Work out the finished part from the listing and answer in its coordinate system (mm). A direction names the side the tool comes from. Give positions to 0.01 mm unless a question says otherwise; leave off trailing zeros. Order: outer loops, then holes, each group sorted by start corner. A loop starts at its lowest first (then second) coordinate and runs counter-clockwise, first axis right, second up. Notation, with made-up numbers: (48.5, 87.25) - (57.5, 87.25) arc R26 cw to (57.5, 122.25) - close; hole circle Ø7 at (29.25, 77). An arc over 180 degrees is marked (long way). Write each question's results on one line, items separated by ' | '.
from build123d import *

# Parameters (mm, degrees)
F0_W     = 19.05
F0_H     = 19.05
F0_W_2   = 15.875
F0_H_2   = 15.875
F1_DEPTH = 40
F3_DEPTH = 9.526
F4_DEPTH = 9.526
F5_R     = 3
F6_DEPTH = 9.526


with BuildPart() as f1:
    # F0 (on Front) → F1 (new body)
    with BuildSketch(Plane.XZ):
        Rectangle(F0_W, F0_H)
        Rectangle(F0_W_2, F0_H_2, mode=Mode.SUBTRACT)
    extrude(amount=F1_DEPTH)

    # F2 (on Top) → F3 (cut, through all)
    with BuildSketch(Plane.XY):
        Polygon((9.525, 0), (-9.525, 0), (-9.525, -19.05), align=None)
    extrude(amount=-F3_DEPTH, mode=Mode.SUBTRACT)

    # F2 (on Top) → F4 (cut, through all)
    with BuildSketch(Plane.XY):
        Polygon((9.525, 0), (-9.525, 0), (-9.525, -19.05), align=None)
    extrude(amount=F4_DEPTH, mode=Mode.SUBTRACT)

    # F5 (on Right) → F6 (cut, through all)
    with BuildSketch(Plane.YZ):
        with Locations((-32.75, 0)):
            Circle(F5_R)
    extrude(amount=-F6_DEPTH, mode=Mode.SUBTRACT)


solid = f1.part
1. Straight lines are drawn through the part: line 1 (X direction, y = -24, z = 0.5) (1 decimal); line 2 (Z direction, x = -8.5, y = -32.75) (3 decimals). For each, find the intervals that lie inside material, in ascending order. Write a range as [from, to].
Answer list:
line 1: [-9.5, -7.9], [7.9, 9.5] | line 2: [-9.525, -3], [3, 9.525]
2. A tool of negligible diameter and unlimited length cuts with its end or side. For faces 1 (the face through (-9, -40, 0)), 2 (the face through (0, -25, 7.938)), 3 (the face through (-8.72, -35.747, 0.132)), from which of +Z, -Z, +X, -X, +Y, -Y can it reach the whole face along a straight path? Write none if from no direction.
Answer list:
face 1: +Z, -Z, +X, -X, -Y | face 2: +Y, -Y | face 3: -X
3. A cutting plane is placed at C-C, the plane z = 0. State how many separate pieces and enclosed holes the cut face has, then the cut area to 3 significant figures.
Answer list:
separate pieces: 3 | enclosed holes: 0 | area: 87.2 mm^2
4. A cutting plane is placed at B-B, the plane x = 0.75. Write down the section's boundary in (y, z) (1 decimal), then the cut area to 3 significant figures.
Answer list:
outline: (-40, -9.5) - (-8.8, -9.5) - (-8.8, -7.9) - (-40, -7.9) - close; (-40, 7.9) - (-8.8, 7.9) - (-8.8, 9.5) - (-40, 9.5) - close | area: 99.1 mm^2
5. Given P1, Ø6, axis at y = -10, z = -3.5, coming from the -X side; P2, Ø9.5, axis at y = -32.75, z = 0, coming from the -X side (3 decimals), each flat-ended and moving along its own axis, determine where each tip first touches the part or whether it passes through.
Answer list:
P1: x = 7.94 | P2: x = -9.525
6. A cutting plane is placed at D-D, the plane y = -32.75. Write down the section's boundary in (x, z) (1 decimal), then the cut area to 3 significant figures.
Answer list:
outline: (-9.5, -9.5) - (9.5, -9.5) - (9.5, 9.5) - (-9.5, 9.5) - (-9.5, 3) - (-7.9, 3) - (-7.9, 7.9) - (7.9, 7.9) - (7.9, -7.9) - (-7.9, -7.9) - (-7.9, -3) - (-9.5, -3) - close | area: 101 mm^2
7. Determine the mould class of faces 4 (the face through (0, -24, -9.525)), 5 (the face through (-7.938, -29, 0)), 6 (the face through (9.525, -20, 0)) for opening direction Z: +Z half, -Z half, draft (parallel to the pull), parting line (faces both ways), or undercut.
Answer list:
face 4: -Z half | face 5: undercut | face 6: draft
